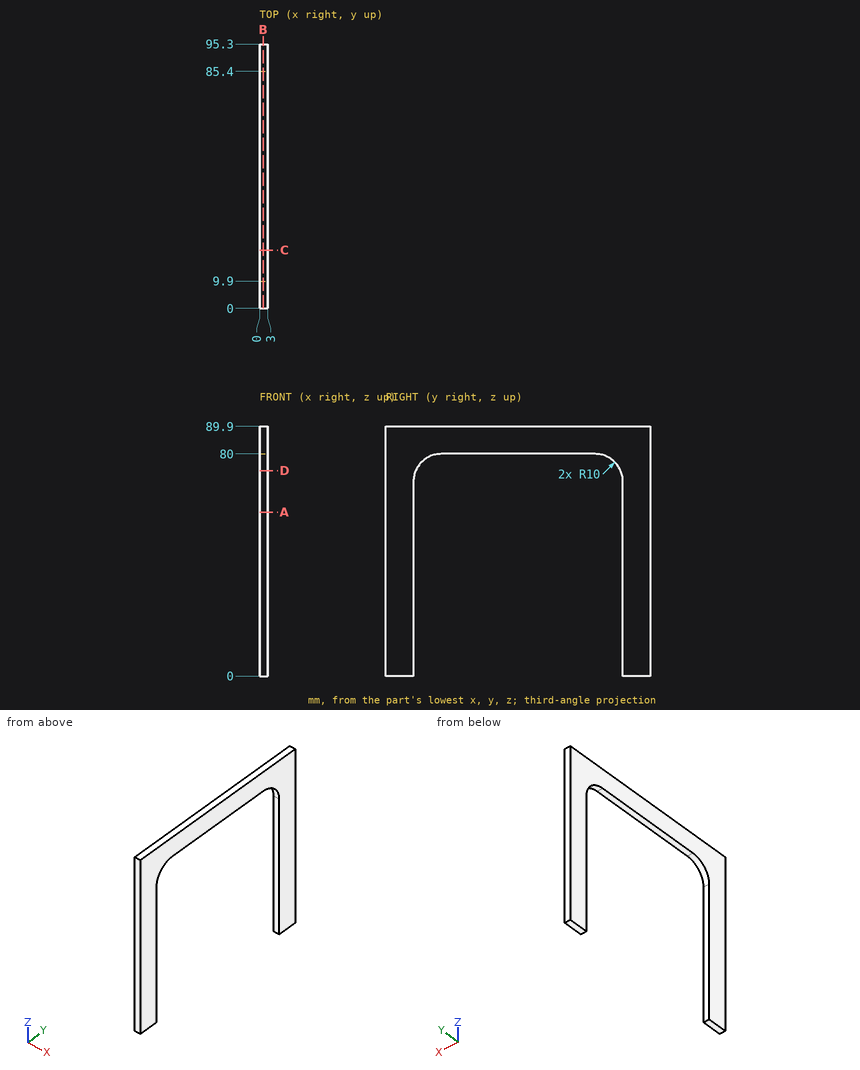
Job drawing, mm, ordinate dimensions from the low corner. One solid piece. Round coordinates to 2 decimals unless told otherwise and drop trailing zeros. Loops run counter-clockwise (first coordinate to the right, second up) from the corner with the lowest first, then second, coordinate; pieces in that order, holes last. Notation, with made-up numbers: (-8, 3) -> (30, 3) arc R12 cw to (30, 13) -> close; hole circle Ø6 at (36, 5.5). An arc over 180 degrees is marked (long way). Use CSV: the item, a comma, the result in double quotes. Start each with the question number.
Q1. Saw through at B-B on x = 1.3. Give the cut face in (y, z).
Q2. Flat gauge pins, fed straight in: pin 1 Ø12 at (y, z) = (83.5, 15.5) entering from -X; pin 2 Ø1.5 at (x, y) = (1.5, 37) entering from -Z; pin 3 Ø4 at (y, z) = (33, 77) entering from +X. Where does each tip first touch, or does it go through?
Q3. Saw through at A-A on z = 59. Give the cut face in (x, y), and give its area (3 significant figures).
Q4. Saw through at C-C on y = 21. Give the cut face in (x, z), and give its area (3 significant figures).
Q5. Drill centre lines: L1, parallel to Y at x = 1.7, z = 59; L2, parallel to Y at x = 0.1, z = 73; L3, parallel to Z at x = 0.35, y = 57.5. Where is each one in solid material? Low to high.
Q6. Saw through at D-D on z = 74. Give the cut face in (x, y), and give its area (3 significant figures).
Solutions:
1,outline,"(0, 0) -> (9.9, 0) -> (9.9, 70) arc R10 cw to (19.9, 80) -> (75.4, 80) arc R10 cw to (85.4, 70) -> (85.4, 0) -> (95.3, 0) -> (95.3, 89.9) -> (0, 89.9) -> close"
2,pin 1,"stops at x = 0"
2,pin 2,"stops at z = 80"
2,pin 3,"passes through"
3,outline,"(0, 0) -> (3, 0) -> (3, 9.9) -> (0, 9.9) -> close; (0, 85.4) -> (3, 85.4) -> (3, 95.3) -> (0, 95.3) -> close"
3,area,"59.4 mm^2"
4,outline,"(0, 80) -> (3, 80) -> (3, 89.9) -> (0, 89.9) -> close"
4,area,"29.7 mm^2"
5,L1,"y = 0 to 9.9, 85.4 to 95.3"
5,L2,"y = 0 to 10.36, 84.94 to 95.3"
5,L3,"z = 80 to 89.9"
6,outline,"(0, 0) -> (3, 0) -> (3, 10.73) -> (0, 10.73) -> close; (0, 84.57) -> (3, 84.57) -> (3, 95.3) -> (0, 95.3) -> close"
6,area,"64.4 mm^2"
